Autodesk Inventor part; units mm, degrees
ref_plane "YZ Plane" through (0, 0, 0) normal (1, 0, 0) x (0, 1, 0)
ref_plane "XZ Plane" through (0, 0, 0) normal (0, 1, 0) x (-1, 0, 0)
ref_plane "XY Plane" through (0, 0, 0) normal (0, 0, 1) x (1, 0, 0)
sketch "Sketch1" plane through (0, 0, 0) normal (0, 1, 0) x (-1, 0, 0)
  line L0 (70, 34) -> (-70, 34)
  line L1 (-70, 34) -> (-70, -34)
  line L2 (-70, -34) -> (70, -34)
  line L3 (70, -34) -> (70, 34)
  line L4 (70, 0) -> (-70, 0) construction
  line L5 (0, 34) -> (0, -34) construction
  line L6 (70, 34) -> (66, 34) construction
  line L7 (66, 34) -> (66, 30) construction
  line L8 (66, 30) -> (70, 30) construction
  line L9 (70, 30) -> (70, 34) construction
  circle A0 centre (66, 30) radius 1.25
  circle A1 centre (66, -30) radius 1.25
  circle A2 centre (-66, 30) radius 1.25
  circle A3 centre (-66, -30) radius 1.25
  point P0 (0, 0)
  point P1 (0, 0)
  dimension "d0" = 68
  dimension "d1" = 140
  dimension "d4" = 4
  dimension "d5" = 4
  dimension "d6" = 2.5
extrude "Extrusion1" add sketch "Sketch1" along normal blind 2
sketch "Sketch2" plane through (0, 2, 0) normal (0, 1, 0) x (1, 0, 0)
  line L0 (-24.1481, -20) -> (24.1481, -20)
  line L1 (24.1481, -20) -> (24.1481, 20)
  line L2 (24.1481, 20) -> (-24.1481, 20)
  line L3 (-24.1481, 20) -> (-24.1481, -20)
  line L4 (-24.1481, 0) -> (24.1481, 0) construction
  line L5 (0, -20) -> (0, 20) construction
  point P0 (0, 0)
  point P1 (0, 0)
  dimension "d7" = 48.2963
  dimension "d8" = 40
extrude "Extrusion2" add sketch "Sketch2" along normal blind 30
sketch "Sketch3" plane through (-24.1481, 2, 20) normal (0, 0, 1) x (1, 0, 0)
  line L0 (0, 0) -> (0, 30)
  line L1 (0, 30) -> (48.2963, 17.059)
  line L2 (48.2963, 0) -> (48.2963, 30)
  line L3 (0, 30) -> (48.2963, 30)
  point P0 (24.1481, -2)
  dimension "d11" = 15
extrude "Extrusion3" cut sketch "Sketch3" against normal up to next
sketch "Sketch5" plane through (-24.1481, 32, 20) normal (0.2588, 0.9659, 0) x (0.9659, -0.2588, 0)
  line L0 (40, 5) -> (10, 5) construction
  line L1 (10, 5) -> (10, 35) construction
  line L2 (10, 35) -> (40, 35) construction
  line L3 (40, 35) -> (40, 5) construction
  line L4 (50, 40) -> (50, 0) construction
  line L5 (50, 20) -> (0, 20) construction
  line L6 (0, 40) -> (0, 0) construction
  line L7 (7.7646, 40) -> (0, 40) construction
  line L8 (7.7646, 0) -> (0, 0) construction
  line L9 (40, 20) -> (10, 20) construction
  circle A0 centre (40, 5) radius 2.5
  circle A1 centre (40, 35) radius 2.5
  circle A2 centre (10, 35) radius 2.5
  circle A3 centre (10, 5) radius 2.5
  point P0 (31.6075, 20)
  point P1 (25, 20)
  dimension "d18" = 30
  dimension "d19" = 30
  dimension "d20" = 5
  dimension "d21" = 5
  dimension "d22" = 5
  dimension "d23" = 5
extrude "Extrusion5" cut sketch "Sketch5" against normal blind 7
sketch "Sketch6" plane through (0, 0, 0) normal (0, -1, 0) x (1, 0, 0)
  line L0 (-24.1481, -20) -> (24.1481, -20)
  line L1 (24.1481, -20) -> (24.1481, 20)
  line L2 (-24.1481, 20) -> (-24.1481, -20)
  line L3 (24.1481, 20) -> (-24.1481, 20)
  line L4 (-7.2444, 7.5) -> (7.2444, 7.5)
  line L5 (7.2444, 7.5) -> (7.2444, -7.5)
  line L6 (7.2444, -7.5) -> (-7.2444, -7.5)
  line L7 (-7.2444, -7.5) -> (-7.2444, 7.5)
  line L8 (0, -7.5) -> (0, 7.5) construction
  point P0 (0, 0)
  point P1 (0, 0)
  dimension "d26" = 14.4889
  dimension "d27" = 15
extrude "Extrusion6" cut sketch "Sketch6" against normal up to next contours L4 L5 L6 L7
properties part number "touchscreen_support"
Geometry check sheet. Reference: the model listing, model coordinates, mm. A direction names the side the tool comes from. Give positions to 0.01 mm unless a question says otherwise; leave off trailing zeros. Loops run counter-clockwise (first coordinate to the right, second up) from the corner with the lowest first, then second, coordinate; pieces in that order, holes last. Notation, with made-up numbers: (29.25, 59) -> (34.25, 59) arc R22 ccw to (34.25, 89) -> close; hole circle Ø7 at (7, -37). An arc over 180 degrees is marked (long way). Answer in a Markdown table with one row per item. Add a question column.
1) Cross-section at C-C on x = -33. Record the boundary of the cut face in (y, z), and give its area (3 significant figures).
2) Gauge pin test, flat ends, axial feed: P1, Ø7.5, axis at y = 20, z = 0.5, coming from the +X side; P2, Ø2, axis at x = -9, y = 12, coming from the +Z side; P3, Ø1.5, axis at x = 66, z = -30, coming from the +Y side; P4, Ø4.5, axis at x = -2.5, y = 20.5, coming from the -Z side. Record the tip position at first contact, or that the pin passes through.
3) Draft check along Y on faces 6 (the face through (-0.34, 25.62, -8.61)), 7 (the face through (14.71, 18.014, -12.782)), 8 (the face through (7.244, 12, 0)), 9 (the face through (12.643, 14.893, -15.035)). Enter one of: pulls with the +Y half, pulls with the -Y half, needs draft (parallel to the pull), parting line crosses it, or undercut.
4) Cross-section at A-A on x = 3. Record the boundary of the cut face in (y, z).
5) Set-up check for faces 1 (the face through (0, 14, -7.5)), 2 (the face through (-24.148, 17, 0)), 3 (the face through (0, 13, -20)), 4 (the face through (0, 13, 20)), 5 (the face through (24.148, 10, 0)): record each of +Z, -Z, +X, -X, +Y, -Y from which the full face is reachable in a straight line by a thin tool's end or side.
6) Material ranges on probe 1 along Z at (x, y) = (66, 1.55); probe 2 along Z at (x, y) = (-6.5, 21); probe 3 along Y at (x, z) = (-48.5, -16), recorded low to high. Write a range as from..to.
7) Cross-section at B-B on y = 9. Record the boundary of the cut face in (x, z).
8) Cross-section at D-D on y = 17.5. State how many separate pieces and enclosed holes the cut face has, and give its area (3 significant figures).
Outcome:
| question | item | result |
|---|---|---|
| 1 | outline | (0, -34) -> (2, -34) -> (2, 34) -> (0, 34) -> close |
| 1 | area | 136 mm^2 |
| 2 | P1 | stops at x = 24.15 |
| 2 | P2 | stops at z = 20 |
| 2 | P3 | passes through |
| 2 | P4 | stops at z = -20 |
| 3 | face 6 | pulls with the +Y half |
| 3 | face 7 | undercut |
| 3 | face 8 | needs draft |
| 3 | face 9 | undercut |
| 4 | outline | (0, -34) -> (2, -34) -> (2, -20) -> (24.73, -20) -> (24.73, -7.5) -> (0, -7.5) -> close; (0, 7.5) -> (24.73, 7.5) -> (24.73, 20) -> (2, 20) -> (2, 34) -> (0, 34) -> close |
| 5 | face 1 | +Y, -Y |
| 5 | face 2 | +Z, -Z, -X, +Y |
| 5 | face 3 | -Z, +X, -X, +Y |
| 5 | face 4 | +Z, +X, -X, +Y |
| 5 | face 5 | +Z, -Z, +X, +Y |
| 6 | probe 1 | z = -34..-31.25, -28.75..28.75, 31.25..34 |
| 6 | probe 2 | z = -20..-7.5, 7.5..20 |
| 6 | probe 3 | y = 0..2 |
| 7 | outline | (-24.15, -20) -> (24.15, -20) -> (24.15, 20) -> (-24.15, 20) -> close; hole (-7.24, -7.5) -> (7.24, -7.5) -> (7.24, 7.5) -> (-7.24, 7.5) -> close |
| 8 | separate pieces | 1 |
| 8 | enclosed holes | 3 |
| 8 | area | 1,670 mm^2 |
